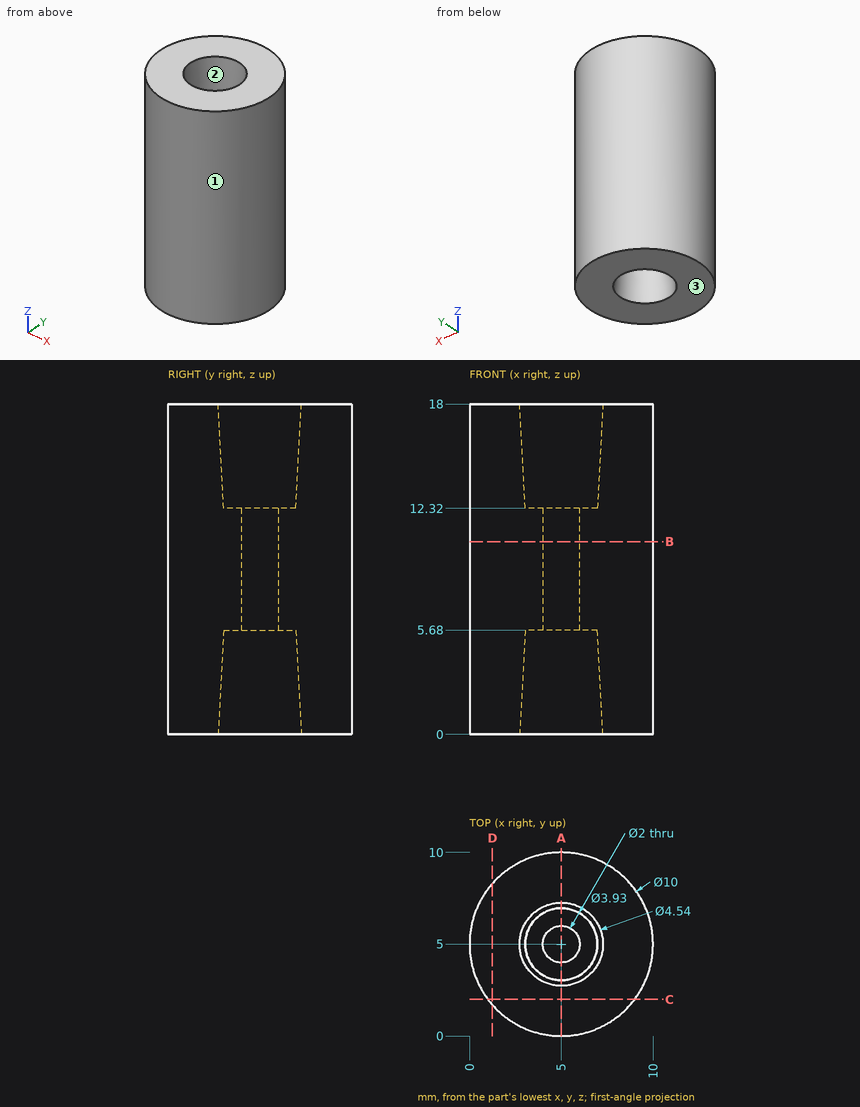
Part print with two shaded views. Sizes in mm from the minimum x, y, z corner. Give positions to 0.01 mm unless a question says otherwise; leave off trailing zeros. Order: outer loops, then holes, each group sorted by start corner. A loop starts at its lowest first (then second) coordinate and runs counter-clockwise, first axis right, second up.
1) Saw through at D-D, the plane x = 1.25. Write the cut outline in (y, z).
2) Wall check: probe 1 along Y at (x, z) = (5, 10); probe 2 along Z at (x, y) = (6.5, 5.5); probe 3 along Y at (x, z) = (5.75, 7.75). Give the ranges that are in metal, low to high.
3) Mould opens along Y. For the marked faces 1, 2 and 3 say: +Y half, -Y half, draft (parallel to the pull), parting line (faces both ways), or undercut.
4) Pin check, flat tips, straight feed: pin 1 (1.5 mm diameter, centred on x = 3.5, y = 6.5, fed in from +Z); pin 2 (1.5 mm diameter, centred on y = 3, z = 9.5, fed in from +X); pin 3 (5 mm diameter, centred on y = 9, z = 5, fed in from -X); pin 4 (1.5 mm diameter, centred on y = 1.5, z = 6, fed in from +X). Stop position of each tip, or through.
5) Saw through at C-C, the plane y = 2. Write the cut outline in (x, z).
6) Saw through at B-B, the plane z = 10.5. Write the cut outline in (x, y), then the cut area to 3 significant figures.
7) Saw through at A-A, the plane x = 5. Write the cut outline in (y, z) (3 decimals), then the cut area to 3 significant figures.
Computed:
1. outline: (1.69, 0) - (8.31, 0) - (8.31, 18) - (1.69, 18) - close
2. probe 1: y = 0 to 4, 6 to 10
2. probe 2: z = 5.68 to 12.32
2. probe 3: y = 0.06 to 4.34, 5.66 to 9.94
3. face 1: parting line
3. face 2: undercut
3. face 3: draft
4. pin 1: stops at z = 18
4. pin 2: stops at x = 9.84
4. pin 3: stops at x = 0.23
4. pin 4: stops at x = 9.18
5. outline: (1, 0) - (9, 0) - (9, 18) - (1, 18) - close
6. outline: circle Ø10 at (5, 5); hole circle Ø2 at (5, 5)
6. area: 75.4 mm2
7. outline: (0, 0) - (2.73, 0) - (3.035, 5.68) - (4, 5.68) - (4, 12.32) - (3.035, 12.32) - (2.73, 18) - (0, 18) - close; (6, 5.68) - (6.965, 5.68) - (7.27, 0) - (10, 0) - (10, 18) - (7.27, 18) - (6.965, 12.32) - (6, 12.32) - close
7. area: 119 mm2
